Source: CAD feature listing. Evaluate the final solid. Frame: model axes, mm. A direction names the side the tool comes from. Give positions to 0.01 mm unless a question says otherwise; leave off trailing zeros. Loops run counter-clockwise (first coordinate to the right, second up) from the corner with the lowest first, then second, coordinate; pieces in that order, holes last. Notation, with made-up numbers: (-4, 4.25) -> (13, 4.25) arc R14 cw to (13, 21.25) -> close; hole circle Ø10 at (-15, 52). An arc over 180 degrees is marked (long way). Return JSON: item names as keys, results as strings. Group by question number.
(1) Access query for faces 1 (the face through (0.14, -5.96, 8.8)), 2 (the face through (0, 1, 0)). Directions: +Z, -Z, +X, -X, +Y, -Y. A direction counts if a zero-diameter tool reaches every point of the face in a straight line with its end or side. Return the directions, or none.
(2) Draft query along Z for faces 3 (the face through (0, 4, 3)), 4 (the face through (10, -4, 2)), 5 (the face through (0, -10, 9)). Return one class per face: released by +Z, released by -Z, zero draft, split by the parting line, or undercut.
(3) Pin query (flat end, axial travel): pin 1 (2.5 mm diameter, centred on x = 0, y = 11.5, fed in from -Z); pin 2 (4 mm diameter, centred on x = 4, z = 8, fed in from -Y); pin 3 (8 mm diameter, centred on x = -4.5, y = 11, fed in from +Z); pin 4 (1 mm diameter, centred on x = -3.5, z = 4.5, fed in from -Y). Return the tip coordinate at first contact, or that it passes through.
(4) Ray query, line 1 (Y direction, x = 0, z = 1.65); line 2 (X direction, y = 11.5, z = 1.45); line 3 (Z direction, x = -3.25, y = -11.5). Return the intervals inside material, ascending. Write a range as from..to.
(5) Cut plane D-D on x = 8. Return loops of the section in (y, z).
(6) Cut plane A-A on y = 11.5. Return loops of the section in (x, z).
(7) Cut plane C-C on z = 2.25. Return loops of the section in (x, y), then the cut area to 3 significant figures.
(8) Cut plane B-B on x = 0. Return loops of the section in (y, z), then the cut area to 3 significant figures.
```python
from build123d import *

# Parameters (mm, degrees)
F1_DEPTH = 10
F2_R     = 5
F4_D     = 3


with BuildPart() as f1:
    # F0 (on Right) → F1 (new body, symmetric)
    with BuildSketch(Plane.YZ):
        Polygon((-11.7573593129, 3), (0, 14.7573593129), (-4.2426406871, 14.7573593129), (-16, 3), (-16, 0), (19, 0), (19, 3), align=None)
    extrude(amount=F1_DEPTH, both=True)

    # F2
    f2_edges = [f1.edges().sort_by_distance(p)[0] for p in [
        (10, 19, 1.5),
        (-10, 19, 1.5),
    ]]
    fillet(f2_edges, radius=F2_R)

    # F4 (through all)
    with Locations(Plane(origin=(0, 0, 0), x_dir=(1, 0, 0), z_dir=(0, 0, -1))):
        with Locations((0, -11.5)):
            Hole(F4_D / 2)


solid = f1.part
```
Answers:
{
 "1": {"face 1": "+X, -X, +Y", "face 2": "-Z, +X, -X, +Y, -Y"},
 "2": {"face 3": "undercut", "face 4": "zero draft", "face 5": "released by +Z"},
 "3": {"pin 1": "through", "pin 2": "y = -13", "pin 3": "z = 3", "pin 4": "y = -15"},
 "4": {"line 1": "-16..10, 13..19", "line 2": "-10..-1.5, 1.5..10", "line 3": "0..3, 3.26..7.5"},
 "5": {"outline": "(-16, 0) -> (18, 0) -> (18, 3) -> (-11.76, 3) -> (0, 14.76) -> (-4.24, 14.76) -> (-16, 3) -> close"},
 "6": {"outline": "(-10, 0) -> (-1.5, 0) -> (-1.5, 3) -> (-10, 3) -> close; (1.5, 0) -> (10, 0) -> (10, 3) -> (1.5, 3) -> close"},
 "7": {"outline": "(-10, -16) -> (10, -16) -> (10, 14) arc R5 ccw to (5, 19) -> (-5, 19) arc R5 ccw to (-10, 14) -> close; hole circle Ø3 at (0, 11.5)", "area": "682 mm²"},
 "8": {"outline": "(-16, 0) -> (10, 0) -> (10, 3) -> (-11.76, 3) -> (0, 14.76) -> (-4.24, 14.76) -> (-16, 3) -> close; (13, 0) -> (19, 0) -> (19, 3) -> (13, 3) -> close", "area": "146 mm²"}
}
